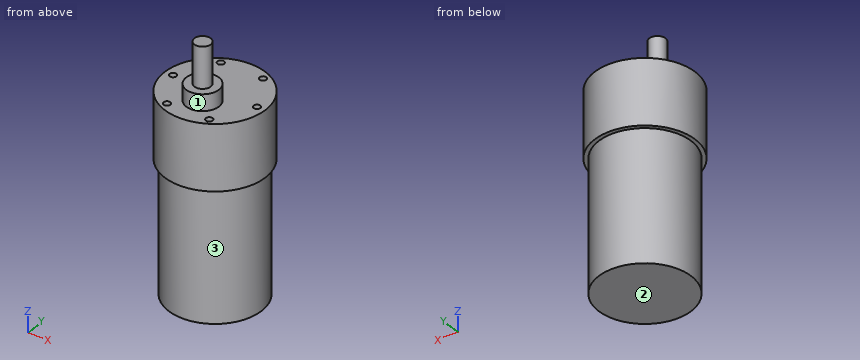
```python
from build123d import *

# Parameters (mm, degrees)
CROQUIS1_R              = 17
SALIENTE_EXTRUIR1_DEPTH = 48
CROQUIS2_R              = 18.5
SALIENTE_EXTRUIR2_DEPTH = 24
CROQUIS3_R              = 6
SALIENTE_EXTRUIR3_DEPTH = 6
CROQUIS4_R              = 3
SALIENTE_EXTRUIR4_DEPTH = 15
CROQUIS5_R              = 1.25
CORTAR_EXTRUIR3_DEPTH   = 14


with BuildPart() as part:
    # Croquis1 → Saliente-Extruir1 (new body)
    with BuildSketch(Plane.XY):
        Circle(CROQUIS1_R)
    extrude(amount=SALIENTE_EXTRUIR1_DEPTH)

    # Croquis2 → Saliente-Extruir2 (add)
    with BuildSketch(Plane.XY.offset(48)):
        Circle(CROQUIS2_R)
    extrude(amount=SALIENTE_EXTRUIR2_DEPTH)

    # Croquis3 → Saliente-Extruir3 (add)
    with BuildSketch(Plane.XY.offset(72)):
        with Locations((0, -6.5)):
            Circle(CROQUIS3_R)
    extrude(amount=SALIENTE_EXTRUIR3_DEPTH)

    # Croquis4 → Saliente-Extruir4 (add)
    with BuildSketch(Plane.XY.offset(78)):
        with Locations((0, -6.5)):
            Circle(CROQUIS4_R)
    extrude(amount=SALIENTE_EXTRUIR4_DEPTH)

    # Croquis5 → Cortar-Extruir3 (cut)
    with BuildSketch(Plane.XY.offset(72)):
        with Locations((-7.75, -14)):
            Circle(CROQUIS5_R)
        with Locations((7.75, -14)):
            Circle(CROQUIS5_R)
        with Locations((-15.4, 0)):
            Circle(CROQUIS5_R)
        with Locations((15.4, 0)):
            Circle(CROQUIS5_R)
        with Locations((-7.75, 14)):
            Circle(CROQUIS5_R)
        with Locations((7.75, 14)):
            Circle(CROQUIS5_R)
    extrude(amount=-CORTAR_EXTRUIR3_DEPTH, mode=Mode.SUBTRACT)


solid = part.part
```
CAD build for the part. Positions are in the model's coordinates, mm. Face numbers are marked on the shaded views. A direction names the side the tool comes from. Round coordinates to 2 decimals unless told otherwise and drop trailing zeros. Loops run counter-clockwise (first coordinate to the right, second up) from the corner with the lowest first, then second, coordinate; pieces in that order, holes last. Notation, with made-up numbers: M 40.5,78.5 L 90.5,78.5 A19 ccw 90.5,115.5 Z; hole C -26,58.25 d1. An arc over 180 degrees is marked long. Return JSON: item names as keys, results as strings. Group by question number.
(1) Tool access for the marked faces 1, 2 and 3: list every direction of +Z, -Z, +X, -X, +Y, -Y with a clear straight run to the whole face (end or side of a thin tool).
(2) Drop flat-ended pins along their axis: P1, Ø1.5, axis at x = -7.75, y = 14, coming from the -Z side; P2, Ø1.2, axis at x = 8, y = 13.5, coming from the +Z side; P3, Ø3, axis at y = 12.5, z = 33.5, coming from the -X side; P4, Ø6, axis at x = 5.5, z = 80, coming from the -Y side. Give the stop position or say it passes through.
(3) Saw through at A-A, the plane x = 15.4. List the corners of the cut face in (y, z).
(4) Saw through at C-C, the plane z = 44.5. List the corners of the cut face in (x, y), and give its area (3 significant figures).
(5) Wall check: probe 1 along Z at (x, y) = (-16, 4); probe 2 along Z at (x, y) = (12.5, -12); probe 3 along Y at (x, z) = (15, 63). Give the ranges that are in metal, low to high. Write a range as [from, to].
(6) Saw through at B-B, the plane y = -6.5. List the corners of the cut face in (x, z).
(7) Saw through at D-D, the plane x = -15.5. List the corners of the cut face in (y, z), and give its area (3 significant figures).
Answer list:
{
 "1": {"face 1": "+Z", "face 2": "-Z, +X, -X, +Y, -Y", "face 3": "-Z"},
 "2": {"P1": "z = 0", "P2": "z = 58", "P3": "x = -12.96", "P4": "y = -11.53"},
 "3": {"outline": "M -10.25,48 L -7.2,48 L -7.2,0 L 7.2,0 L 7.2,48 L 10.25,48 L 10.25,72 L 1.25,72 L 1.25,58 L -1.25,58 L -1.25,72 L -10.25,72 Z"},
 "4": {"outline": "C 0,0 d34", "area": "908 mm2"},
 "5": {"probe 1": "[0, 72]", "probe 2": "[48, 72]", "probe 3": "[-10.83, -1.18], [1.18, 10.83]"},
 "6": {"outline": "M -17.32,48 L -15.71,48 L -15.71,0 L 15.71,0 L 15.71,48 L 17.32,48 L 17.32,72 L 6,72 L 6,78 L 3,78 L 3,93 L -3,93 L -3,78 L -6,78 L -6,72 L -17.32,72 Z"},
 "7": {"outline": "M -10.1,48 L -6.98,48 L -6.98,0 L 6.98,0 L 6.98,48 L 10.1,48 L 10.1,72 L 1.25,72 L 1.25,58 L -1.25,58 L -1.25,72 L -10.1,72 Z", "area": "1,120 mm2"}
}
